from build123d import *

# Parameters (mm, degrees)
SKETCH1_W           = 8.466666667
SKETCH1_H           = 3.175
BOSS_EXTRUDE1_DEPTH = 5.55625
FILLET1_R           = 0.254


with BuildPart() as part:
    # Sketch1 → Revolve1 (revolve)
    with BuildSketch(Plane.XY, mode=Mode.PRIVATE) as revolve1_sk:
        with Locations((4.233333334, 1.5875)):
            Rectangle(SKETCH1_W, SKETCH1_H)
    revolve(revolve1_sk.sketch.rotate(Axis((-10.583333333, 0, 0), (1, 0, 0)), 90), axis=Axis((-10.583333333, 0, 0), (1, 0, 0)))

    # Sketch2 → Boss-Extrude1 (add)
    with BuildSketch(Plane.ZY):
        Polygon((-5.55625, -3.182294901), (-5.55625, 3.182294901), (0, 6.2865), (5.55625, 3.182294901), (5.55625, -3.182294901), (0, -6.2865), align=None)
    extrude(amount=BOSS_EXTRUDE1_DEPTH)

    # Fillet1
    fillet1_edges = [part.edges().sort_by_distance(p)[0] for p in [
        (0, 0, -3.175),
    ]]
    fillet(fillet1_edges, radius=FILLET1_R)


solid = part.part
For this review, take the finished solid that the model builds, in its own axes (mm). A direction names the side the tool comes from. Coordinates: 2 decimals unless noted, no trailing zeros. Loops run counter-clockwise (first coordinate to the right, second up) from the corner with the lowest first, then second, coordinate; pieces in that order, holes last. Notation, with made-up numbers: (37, -35.5) - (69, -35.5) arc R24 cw to (69, -23.5) - close; hole circle Ø3 at (-5.75, 59.5). An arc over 180 degrees is marked (long way). Use a Markdown table: item, result. Add a question column.
Item 1: Insertion check: pin 1 Ø2 at (x, y) = (6.5, -2) entering from -Z; pin 2 Ø5 at (x, y) = (6, 2.5) entering from +Z (3 decimals); pin 3 Ø3 at (y, z) = (5, -2.5) entering from +X. Each pin has a flat end and moves straight along its axis. Give the tip position at first contact, or say it passes through.
Item 2: We need section C-C (x = 4.5). Give the boundary of the cut face in (y, z) (3 decimals).
Item 3: We need section A-A (x = -2.75). Give the boundary of the cut face in (y, z), and give its area (3 significant figures).
Item 4: Tool access review of faces 1 (the face through (8.467, 0, 0)), 2 (the face through (4.42, 1.93, -2.52)): name each direction out of +Z, -Z, +X, -X, +Y, -Y from which nothing blocks a thin tool from reaching the whole face with its end or side.
Item 5: We need section D-D (y = 5.25). Give the boundary of the cut face in (x, z), and give its area (3 significant figures).
Item 6: For line 1 (X direction, y = 0.5, z = -3.5); line 2 (Z direction, x = 6, y = 2.75); line 3 (Y direction, x = 2.5, z = -0.25), list the stretches that pass through material, from the lowest coordinate up.
Item 7: We need section B-B (y = 0). Give the boundary of the cut face in (x, z) (3 decimals).
Results list:
| question | item | result |
|---|---|---|
| 1 | pin 1 | stops at z = -3.01 |
| 1 | pin 2 | stops at z = 3.175 |
| 1 | pin 3 | stops at x = 0 |
| 2 | outline | circle Ø6.35 at (0, 0) |
| 3 | outline | (-6.29, 0) - (-3.18, -5.56) - (3.18, -5.56) - (6.29, 0) - (3.18, 5.56) - (-3.18, 5.56) - close |
| 3 | area | 105 mm^2 |
| 4 | face 1 | +Z, -Z, +X, +Y, -Y |
| 4 | face 2 | +X |
| 5 | outline | (-5.56, -1.86) - (0, -1.86) - (0, 1.86) - (-5.56, 1.86) - close |
| 5 | area | 20.6 mm^2 |
| 6 | line 1 | x = -5.56 to 0 |
| 6 | line 2 | z = -1.59 to 1.59 |
| 6 | line 3 | y = -3.17 to 3.17 |
| 7 | outline | (-5.556, -5.556) - (0, -5.556) - (0, -3.429) arc R0.254 cw to (0.254, -3.175) - (8.467, -3.175) - (8.467, 3.175) - (0.254, 3.175) arc R0.254 cw to (0, 3.429) - (0, 5.556) - (-5.556, 5.556) - close |
